Source: CAD feature listing. Evaluate the final solid. Frame: model axes, mm. Face numbers are marked on the shaded views. Round coordinates to 2 decimals unless told otherwise and drop trailing zeros. Order: outer loops, then holes, each group sorted by start corner. A loop starts at its lowest first (then second) coordinate and runs counter-clockwise, first axis right, second up. Notation, with made-up numbers: (44.25, 42) - (102.25, 42) arc R17 cw to (102.25, 51) - close; hole circle Ø7 at (58.25, -13). An arc over 180 degrees is marked (long way). Put each result on its own line as item: value. Start each with the question number.
1) Section B-B on z = 26. Output: boundary loops of the cut face in (x, y).
2) Section C-C on y = 0. Output: boundary loops of the cut face in (x, z), then the cut area to 3 significant figures.
3) Mould query, pull axis X, two halves, no side actions, for the marked faces 1, 2 and 3. Classes: +X half, -X half, draft (parallel to the pull), parting line (faces both ways), or undercut.
4) Section A-A on x = 0. Output: boundary loops of the cut face in (y, z).
5) Line query: probe 1 along Z at (x, y) = (14, 20); probe 2 along Y at (x, z) = (10, 8); probe 3 along Y at (x, z) = (0, 26). Output: solid intervals per line, ascending. Write a range as [from, to].
6) Contact query for flat-ended pins moving along their axis: P1, Ø6.5, axis at y = -20, z = 32, coming from the +X side; P2, Ø7, axis at y = 20, z = 8, coming from the +X side; P3, Ø3.5, axis at y = 20, z = 32, coming from the +X side. Output: stop coordinate, or through.
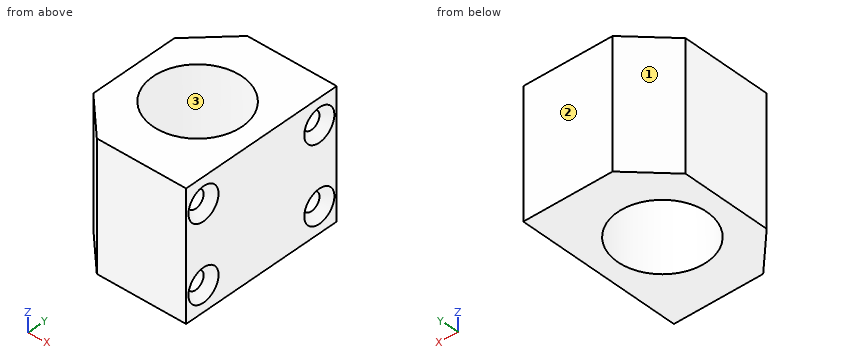
```python
from build123d import *

# Parameters (mm, degrees)
BOSS_EXTRUDE1_DEPTH                                  = 40
SKETCH2_R                                            = 14
CUT_EXTRUDE1_DEPTH                                   = 40
CSK_FOR_M5_COUNTERSUNK_RAISED_HEAD_SCREW_D           = 5.5
CSK_FOR_M5_COUNTERSUNK_RAISED_HEAD_SCREW_DEPTH       = 12
CSK_FOR_M5_COUNTERSUNK_RAISED_HEAD_SCREW_CSINK_D     = 10.4
CSK_FOR_M5_COUNTERSUNK_RAISED_HEAD_SCREW_CSINK_ANGLE = 90
CSK_FOR_M5_COUNTERSUNK_RAISED_HEAD_SCREW_TIP         = 1.652366702


with BuildPart() as part:
    # Sketch1 → Boss-Extrude1 (new body)
    with BuildSketch(Plane.XY):
        Polygon((-20, -14), (-8, -26), (20, -26), (20, 26), (-8, 26), (-20, 14), align=None)
    extrude(amount=BOSS_EXTRUDE1_DEPTH)

    # Sketch2 → Cut-Extrude1 (cut)
    with BuildSketch(Plane.XY.offset(40)):
        Circle(SKETCH2_R)
    extrude(amount=-CUT_EXTRUDE1_DEPTH, mode=Mode.SUBTRACT)

    # CSK for M5 Countersunk Raised Head Screw1
    with Locations(Plane(origin=(20, 0, 0), x_dir=(0, 0, -1), z_dir=(1, 0, 0))):
        with Locations((-32, 20), (-8, 20), (-8, -20), (-32, -20)):
            CounterSinkHole(CSK_FOR_M5_COUNTERSUNK_RAISED_HEAD_SCREW_D / 2, CSK_FOR_M5_COUNTERSUNK_RAISED_HEAD_SCREW_CSINK_D / 2, depth=CSK_FOR_M5_COUNTERSUNK_RAISED_HEAD_SCREW_DEPTH, counter_sink_angle=CSK_FOR_M5_COUNTERSUNK_RAISED_HEAD_SCREW_CSINK_ANGLE)
            with Locations((0, 0, -(CSK_FOR_M5_COUNTERSUNK_RAISED_HEAD_SCREW_DEPTH + CSK_FOR_M5_COUNTERSUNK_RAISED_HEAD_SCREW_TIP / 2))):  # 118° drill point
                Cone(0, CSK_FOR_M5_COUNTERSUNK_RAISED_HEAD_SCREW_D / 2, CSK_FOR_M5_COUNTERSUNK_RAISED_HEAD_SCREW_TIP, mode=Mode.SUBTRACT)


solid = part.part
```
Answer sheet:
1. outline: (-20, -14) - (-8, -26) - (20, -26) - (20, 26) - (-8, 26) - (-20, 14) - close; hole circle Ø28 at (0, 0)
2. outline: (-20, 0) - (-14, 0) - (-14, 40) - (-20, 40) - close; (14, 0) - (20, 0) - (20, 40) - (14, 40) - close
2. area: 480 mm^2
3. face 1: -X half
3. face 2: draft
3. face 3: undercut
4. outline: (-26, 0) - (-14, 0) - (-14, 40) - (-26, 40) - close; (14, 0) - (26, 0) - (26, 40) - (14, 40) - close
5. probe 1: [0, 5.25], [10.75, 29.25], [34.75, 40]
5. probe 2: [-26, -22.75], [-17.25, -9.8], [9.8, 17.25], [22.75, 26]
5. probe 3: [-26, -14], [14, 26]
6. P1: x = 18.05
6. P2: x = 18.3
6. P3: x = 7.4
